Could you check a few things on this model? Use its own coordinates, in mm. A direction names the side the tool comes from. Round coordinates to 2 decimals unless told otherwise and drop trailing zeros. Write each loop counter-clockwise with the first axis right and the second up, starting at its lowest first coordinate (ties: lowest second). Pieces come first, ordered by that corner, then holes. Notation, with made-up numbers: M 50.25,39 L 78.25,39 A18 ccw 78.25,65 Z; hole C -25,72.25 d8. An arc over 180 degrees is marked long. One line per question, with ' | ' between items. Start each with the question number.
```python
from build123d import *

# Parameters (mm, degrees)
SKETCH1_R           = 6.5
BOSS_EXTRUDE1_DEPTH = 21
BOSS_EXTRUDE2_START = -50
SKETCH3_W           = 55
SKETCH3_H           = 21
BOSS_EXTRUDE2_DEPTH = 2
LPATTERN1_COUNT     = 4
LPATTERN1_PITCH     = 8
SKETCH4_R           = 27.5
SKETCH4_R_2         = 7.5
BOSS_EXTRUDE3_DEPTH = 21
SWEEP1_START        = -27.5
SWEEP1_DEPTH        = 55
FILLET1_R           = 3
CUT_EXTRUDE1_START  = 21
CUT_EXTRUDE1_DEPTH  = 21
RIB4_REACH          = 169.295
SKETCH9_WALL_W      = 370.356888496
SKETCH9_WALL_H      = 5


# Read off the part's stored shape, not the designer's step: Sweep1
with BuildPart() as part:
    # Sketch1 → Boss-Extrude1 (new body)
    with BuildSketch(Plane(origin=(0, 0, 0), x_dir=(1, 0, 0), z_dir=(0, 1, 0))):
        with BuildLine():
            Line((0, 27.5), (-80, 27.5))
            Line((-80, 27.5), (-80, -27.5))
            Line((-80, -27.5), (0, -27.5))
            ThreePointArc((0, -27.5), (27.5, 0), (0, 27.5))
        make_face()
        with Locations(Location((0, 0, 0), (0, 0, 90))):
            Circle(SKETCH1_R, mode=Mode.SUBTRACT)
    extrude(amount=BOSS_EXTRUDE1_DEPTH)


with BuildPart() as body_2:
    # Sketch3 → Boss-Extrude2 (new body)
    with BuildSketch(Plane(origin=(0, 0, 0), x_dir=(0, 0, -1), z_dir=(1, 0, 0)).offset(BOSS_EXTRUDE2_START)):
        with BuildLine():
            Line((-33, -15.5), (33, -15.5))
            ThreePointArc((33, -15.5), (40.071067812, -12.571067812), (43, -5.5))
            Line((43, -5.5), (43, 26.5))
            ThreePointArc((43, 26.5), (40.071067812, 33.571067812), (33, 36.5))
            Line((33, 36.5), (-33, 36.5))
            ThreePointArc((-33, 36.5), (-40.071067812, 33.571067812), (-43, 26.5))
            Line((-43, 26.5), (-43, -5.5))
            ThreePointArc((-43, -5.5), (-40.071067812, -12.571067812), (-33, -15.5))
        make_face()
        with Locations((0, 10.5)):
            Rectangle(SKETCH3_W, SKETCH3_H, mode=Mode.SUBTRACT)
    boss_extrude2 = extrude(amount=BOSS_EXTRUDE2_DEPTH)


with BuildPart() as part_1:
    add(part.part)

    # LPattern1: Boss-Extrude2 ×4
    with Locations(*[(-i * LPATTERN1_PITCH, 0, 0) for i in range(1, LPATTERN1_COUNT)]):
        add(boss_extrude2)



with BuildPart() as body_3:
    # Sketch4 → Boss-Extrude3 (new body)
    with BuildSketch(Plane(origin=(0, 10, 0), x_dir=(1, 0, 0), z_dir=(0, 1, 0))):
        with Locations(Location((-130, 0, 0), (0, 0, 90))):
            Circle(SKETCH4_R)
        with Locations(Location((-130, 0, 0), (0, 0, 90))):
            Circle(SKETCH4_R_2, mode=Mode.SUBTRACT)
    extrude(amount=BOSS_EXTRUDE3_DEPTH)


with BuildPart() as part_2:
    add(part_1.part)

    add(body_3.part)  # Sweep1 merges body 3
    # Sweep1 outline → Sweep1 (add)
    with BuildSketch(Plane.XY.offset(SWEEP1_START)):
        with BuildLine():
            Line((-80, 0), (-80, 21))
            add(Edge.make_bspline(
                [(-80, 21), (-86.827647421, 20.344373746), (-93.439203359, 22.931124684), (-105.876424342, 28.26148667), (-111.667729409, 30.999999996), (-119.254055637, 31)],
                knots=[0, 0, 0, 0, 0.5, 0.5, 1, 1, 1, 1], degree=3))
            Line((-119.254055637, 31), (-119.254055637, 10))
            add(Edge.make_bspline(
                [(-80, 0), (-86.827647421, -0.655626254), (-93.439203359, 1.931124684), (-105.876424342, 7.26148667), (-111.667729409, 9.999999996), (-119.254055637, 10)],
                knots=[0, 0, 0, 0, 0.5, 0.5, 1, 1, 1, 1], degree=3))
        make_face()
    extrude(amount=SWEEP1_DEPTH)

    # Fillet1
    # the kernel refuses this fillet: 3 mm, written as the material it takes off along each edge
    with BuildSketch(Plane(origin=(-119.254055637, 38.218973628, -27.5), x_dir=(0, 0, 1), z_dir=(0, -1, 0))) as fillet1_piece_1_section:
        with BuildLine():
            CenterArc((3, -2.887589451), FILLET1_R, 105.734249822, 74.265750178)
            Line((0, -2.887589451), (-0.06, -2.887589451))
            Line((-0.06, -2.887589451), (-0.06, 0))
            Line((-0.06, 0), (0, 0.06))
            ThreePointArc((0, 0.06), (1.093236198, 0.06), (2.170201844, 0.057751789))
            Line((2.170201844, 0.057751789), (2.186472396, 0))
        make_face()
    fillet1_piece_1 = extrude(amount=35.437947255, mode=Mode.PRIVATE)
    fillet1_piece_1 = fillet1_piece_1 - Plane(origin=(-130, 20.5, 0), x_dir=(0, 0, -1), z_dir=(0, -1, 0)) * Cylinder(27.5, 83, mode=Mode.PRIVATE)
    add(fillet1_piece_1, mode=Mode.SUBTRACT)
    with BuildSketch(Plane(origin=(-119.254055637, 38.218973628, 27.5), x_dir=(0, 0, -1), z_dir=(0, -1, 0))) as fillet1_piece_2_section:
        with BuildLine():
            CenterArc((3, 2.887589451), FILLET1_R, 180, 74.265750178)
            Line((0, 2.887589451), (-0.06, 2.887589451))
            Line((-0.06, 2.887589451), (-0.06, 0))
            Line((-0.06, 0), (0, -0.06))
            ThreePointArc((0, -0.06), (1.093236198, -0.06), (2.170201844, -0.057751789))
            Line((2.170201844, -0.057751789), (2.186472396, 0))
        make_face()
    fillet1_piece_2 = extrude(amount=35.437947255, mode=Mode.PRIVATE)
    fillet1_piece_2 = fillet1_piece_2 - Plane(origin=(-130, 20.5, 0), x_dir=(0, 0, -1), z_dir=(0, -1, 0)) * Cylinder(27.5, 83, mode=Mode.PRIVATE)
    add(fillet1_piece_2, mode=Mode.SUBTRACT)

    # Sketch7 → Cut-Extrude1 (cut)
    with BuildSketch(Plane.XZ.offset(-10).offset(CUT_EXTRUDE1_START)):
        with BuildLine():
            ThreePointArc((-119.254055637, 25.313527604), (-157.5, 0), (-119.254055637, -25.313527604))
            ThreePointArc((-119.254055637, -25.313527604), (-102.5, 0), (-119.254055637, 25.313527604))
        make_face()
    extrude(amount=-CUT_EXTRUDE1_DEPTH, mode=Mode.SUBTRACT)


with BuildPart() as body_2_1:
    add(body_2.part)

    # Combine1: union part
    add(part_2.part)

    # Sketch9 wall → Rib4 (add, up to next)
    with BuildSketch(Plane(origin=(-33, 28.75, 0), x_dir=(0.888425906857, -0.459020051876, 0), z_dir=(0.459020051876, 0.888425906857, 0)), mode=Mode.PRIVATE) as rib4_sk1:
        Rectangle(SKETCH9_WALL_W, SKETCH9_WALL_H)
    rib4_tool1 = extrude(rib4_sk1.sketch, amount=-RIB4_REACH, mode=Mode.PRIVATE) - body_2_1.part
    add(rib4_tool1.solids().sort_by_distance((-33, 28.75, 0))[0])


solid = body_2_1.part
```
1. Suppose I cut it at B-B (x = -130). Write out the boundary of the cut face in (y, z), and give its area (3 significant figures).
2. I'm going to push flat-ended pins straight in: P1, Ø1.8, axis at x = -68, z = -0.5, coming from the -Y side; P2, Ø5, axis at y = 5.5, z = -2.5, coming from the +X side; P3, Ø5, axis at x = -77.5, z = -1, coming from the +Y side. Where does each tip first touch, or does it pass through?
3. Suppose I cut it at A-A (z = 29.5). Write out the boundary of the cut face in (x, y), and give its area (3 significant figures).
4. Suppose I cut it at C-C (y = 12). Count the separate pieces of the cut face and the enclosed holes in it, and give its area (3 significant figures).
5. If we mould it in two halves opening along Z, with no side actions, what happens to faces 6 (the face through (-65.01, -12.65, -39.99)), 7 (the face through (-11, 0, 0)), 8 (the face through (-137.436, 20.353, 0.976))? For each: released by +Z, released by -Z, zero draft, split by the parting line, or undercut.
6. Which directions (+Z, -Z, +X, -X, +Y, -Y) give clear straight access to the entire face, cutting with the end or side of a thin tool? Please do faces 1 (the face through (-53, 10, -27.5)), 2 (the face through (-95, 15, -27.5)), 3 (the face through (-38, 27, -2.5)), 4 (the face through (-69, 0, 0)), 5 (the face through (-124, 31, -6)).
7. Suppose I cut it at D-D (y = -8.5). Write out the boundary of the cut face in (x, z).
8. I need wall thicknesses on line 1 along X through (y, z) = (13, 38.5); line 2 along X through (y, z) = (15, 0); line 3 along Z through (x, y) = (-130, 25). Which ranges of each line are inside material? Lowest first, please. Write a range as from..to.
Computed:
1) outline: M 10,-27.5 L 31,-27.5 L 31,-7.5 L 10,-7.5 Z; M 10,7.5 L 31,7.5 L 31,27.5 L 10,27.5 Z | area: 840 mm²
2) P1: stops at y = 0 | P2: stops at x = 27.5 | P3: stops at y = 21
3) outline: M -74,-15.5 L -72,-15.5 L -72,36.5 L -74,36.5 Z; M -66,-15.5 L -64,-15.5 L -64,36.5 L -66,36.5 Z; M -58,-15.5 L -56,-15.5 L -56,36.5 L -58,36.5 Z; M -50,-15.5 L -48,-15.5 L -48,36.5 L -50,36.5 Z | area: 416 mm²
4) separate pieces: 1 | enclosed holes: 2 | area: 9,450 mm²
5) face 6: released by -Z | face 7: zero draft | face 8: undercut
6) face 1: -Z, +Y, -Y | face 2: -Z, -X, +Y, -Y | face 3: -Z, +X, +Y | face 4: +Z, -Z, -Y | face 5: +Z, -Z, -X, +Y
7) outline: M -74,-42.54 L -72,-42.54 L -72,42.54 L -74,42.54 Z; M -66,-42.54 L -64,-42.54 L -64,42.54 L -66,42.54 Z; M -58,-42.54 L -56,-42.54 L -56,42.54 L -58,42.54 Z; M -50,-42.54 L -48,-42.54 L -48,42.54 L -50,42.54 Z
8) line 1: x = -74..-72, -66..-64, -58..-56, -50..-48 | line 2: x = -157.5..-137.5, -122.5..-6.5, 6.5..27.5 | line 3: z = -27.5..-7.5, 7.5..27.5
